Read the model definition and answer for the solid it produces. Units are mm, in the model's axes. Face numbers are marked on the shaded views. A direction names the side the tool comes from. Give positions to 0.01 mm unless a question says otherwise; leave off trailing zeros. Loops run counter-clockwise (first coordinate to the right, second up) from the corner with the lowest first, then second, coordinate; pieces in that order, holes last. Notation, with made-up numbers: (89, -24) - (146, -24) arc R22 cw to (146, 3) - close; hole circle Ø6 at (-26.75, -31). An arc over 180 degrees is marked (long way). Put each result on its own line as item: value. Start each with the question number.
1. A cutting plane is placed at B-B, the plane x = 10.25. Determine the outline of the cut face in (y, z).
2. Given pin 1 Ø5.5 at (x, y) = (-1, -1) entering from -Z; pin 2 Ø6 at (y, z) = (-3.5, -9) entering from +X; pin 3 Ø2 at (y, z) = (-6, -18.5) entering from +X, each flat-ended and moving along its own axis, determine where each tip first touches the part or whether it passes through.
3. A cutting plane is placed at A-A, the plane z = -3.25. Determine the outline of the cut face in (x, y), plus the area to 3 significant figures.
4. A cutting plane is placed at C-C, the plane z = -17.25. Determine the outline of the cut face in (x, y), plus the area to 3 significant figures.
5. Consider L1, parallel to Z at x = 6.25, y = -9.75; L2, parallel to Y at x = 0, z = 3; L3, parallel to Z at x = -5.5, y = 7.25. Determine where each line is inside the solid, lowest interval first. Write a range as from..to.
6. For the marked faces 1, 2 and 3, determine the directions among +Z, -Z, +X, -X, +Y, -Y from which every point of the face is accessible in a straight line to the end or side of a thin tool.
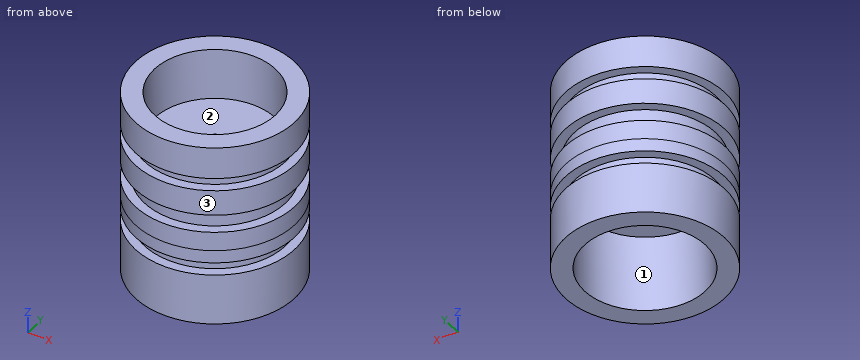
Autodesk Inventor part; units mm, degrees
ref_plane "Work Plane2" through (0, 0, -14) normal (0, 0, -1) x (-1, 0, 0)
ref_plane "Work Plane3" through (0, 0, 1.8) normal (0, 0, 1) x (1, 0, 0)
ref_plane "YZ Plane" through (0, 0, 0) normal (1, 0, 0) x (0, 1, 0)
sketch "Sketch1" plane through (0, 0, 0) normal (0, 0, 1) x (1, 0, 0)
  circle A0 centre (0, 0) radius 0.5
  circle A1 centre (0, 0) radius 8.1639
  point P0 (0, 0)
extrude "Extrusion1" add sketch "Sketch1" along normal blind 9.8
ref_plane "Work Plane1" through (0, 0, -10) normal (0, 0, 1) x (1, 0, 0)
sketch "Sketch2" plane through (0, 0, -10) normal (0, 0, 1) x (1, 0, 0)
  line L0 (5, 5) -> (-5, 5)
  arc A0 (-5, 5) -> (-6, 4) centre (-5, 4) ccw
  line L1 (-6, 4) -> (-6, -4)
  arc A1 (-6, -4) -> (-5, -5) centre (-5, -4) ccw
  line L2 (-5, -5) -> (5, -5)
  arc A2 (5, -5) -> (6, -4) centre (5, -4) ccw
  line L3 (6, -4) -> (6, 4)
  arc A3 (6, 4) -> (5, 5) centre (5, 4) ccw
  circle A4 centre (3.5, 2.5) radius 1.75
  circle A5 centre (-3.5, -2.5) radius 1.75
  circle A6 centre (4.5, 0) radius 0.625
  circle A7 centre (-4.5, 0) radius 0.625
  circle A8 centre (0, 0) radius 2
  line L4 (0, 0) -> (5.8769, -4.8974)
  line L5 (5.8769, -4.8974) -> (7.0292, -5.8577)
  circle A9 centre (0, 0) radius 9.15
  circle A10 centre (0, 0) radius 8.1639
  circle A11 centre (0, 0) radius 13.1
  line L6 (3.0438, -10.097) -> (-9.0477, 9.4736)
  line L7 (-6.9043, 6.0044) -> (-9.0477, 9.4736)
  line L8 (3.0438, -10.097) -> (-5, 4)
  line L9 (-5, 4) -> (-4.2491, 2.684)
  point P0 (0, 0)
  dimension "d3" = 26.2
  dimension "d2" = 1.5
  dimension "d4" = 18.3
extrude "Extrusion2" add sketch "Sketch2" against normal blind 9 contours A9 L8 L6 | A11
sketch "Sketch3" plane through (0, 0, -10) normal (0, 0, 1) x (1, 0, 0)
  arc A0 (0.8877, 1.2091) -> (1.103, -1.0166) centre (0, 0) ccw
  line L0 (0.8877, 1.2091) -> (1.103, -1.0166)
  circle A1 centre (0, 0) radius 13.1
  circle A2 centre (0, 0) radius 9.15
  circle A3 centre (0, 0) radius 8.1639
  circle A4 centre (0, 0) radius 0.5
  point P0 (0, 0)
extrude "Extrusion3" add sketch "Sketch3" along normal up to surface (19.8 mm away) contours A1 | A2 | A3
sketch "Sketch4" plane through (0, 0, 9.8) normal (0, 0, 1) x (1, 0, 0)
  circle A0 centre (0, 0) radius 13.1
  circle A1 centre (0, 0) radius 0.5
  point P0 (0, 0)
extrude "Extrusion4" add sketch "Sketch4" against normal blind 10 contours A1
sketch "Sketch5" plane through (0, 0, 9.8) normal (0, 0, 1) x (1, 0, 0)
  circle A0 centre (0, 0) radius 13.1
  point P0 (0, 0)
extrude "Extrusion5" add sketch "Sketch5" against normal up to surface (9.8 mm away)
sketch "Sketch6" plane through (0, 0, -0.2) normal (0, 0, -1) x (-1, 0, 0)
  circle A0 centre (0, 0) radius 0.5
  point P0 (0, 0)
extrude "Extrusion6" cut sketch "Sketch6" against normal up to surface (0.2 mm away)
sketch "Sketch8" plane through (0, 0, 9.8) normal (0, 0, 1) x (1, 0, 0)
  circle A0 centre (0, 0) radius 13.1
  point P0 (0, 0)
extrude "Extrusion7" cut sketch "Sketch8" against normal blind 3
sketch "Sketch10" plane through (0, 0, -19) normal (0, 0, -1) x (-1, 0, 0)
  circle A0 centre (0, 0) radius 13.1
  circle A1 centre (0, 0) radius 9.15
  circle A2 centre (0, 0) radius 12.5
  line L0 (-12.5, 0) -> (-9.15, 0)
  circle A3 centre (0, 0) radius 9.15
  line L1 (-9.15, 0) -> (-10.825, 0)
  circle A4 centre (0, 0) radius 10.825
  point P0 (0, 0)
  dimension "d18" = 25
extrude "Extrusion8" cut sketch "Sketch10" against normal up to surface (9 mm away)
extrude "Extrusion9" cut sketch "Sketch10" against normal through all contours A0
sketch "Sketch11" plane through (0, 0, -19) normal (0, 0, -1) x (-1, 0, 0)
  circle A0 centre (0, 0) radius 10.825
  line L0 (-0.8877, 1.2091) -> (-1.103, -1.0166)
  arc A1 (-1.103, -1.0166) -> (-0.8877, 1.2091) centre (0, 0) ccw
  circle A2 centre (0, 0) radius 10.825
  circle A3 centre (0, 0) radius 12.5
  line L1 (-12.5, 0) -> (-9.5, 0)
  circle A4 centre (0, 0) radius 9.5
  point P0 (0, 0)
  dimension "d23" = 3
extrude "Extrusion10" add sketch "Sketch11" against normal up to surface (9 mm away) contours A0
sketch "Sketch12" plane through (0, 0, 6.8) normal (0, 0, 1) x (1, 0, 0)
  circle A0 centre (0, 0) radius 12.5
  circle A1 centre (0, 0) radius 9.5
  line L0 (0.8877, 1.2091) -> (1.103, -1.0166)
  arc A2 (0.8877, 1.2091) -> (1.103, -1.0166) centre (0, 0) ccw
  point P0 (0, 0)
extrude "Extrusion11" cut sketch "Sketch12" against normal blind 8 contours A1 | L0 A2
sketch "Sketch13" plane through (0, 0, -1.2) normal (0, 0, 1) x (1, 0, 0)
  line L0 (1.103, -1.0166) -> (0.8877, 1.2091)
  arc A0 (0.8877, 1.2091) -> (1.103, -1.0166) centre (0, 0) ccw
  circle A1 centre (0, 0) radius 9.5
  circle A2 centre (0, 0) radius 11.0657
  circle A3 centre (0, 0) radius 9.5
  circle A4 centre (0, 0) radius 12.5
  point P0 (0, 0)
extrude "Extrusion12" cut sketch "Sketch13" against normal up to surface (8.8 mm away) contours A4
sketch "Sketch14" plane through (0, 0, -10) normal (0, 0, 1) x (1, 0, 0)
  circle A0 centre (0, 0) radius 11.0657
  circle A1 centre (0, 0) radius 12.5
  point P0 (0, 0)
extrude "Extrusion13" add sketch "Sketch14" along normal blind 3
sketch "Sketch15" plane through (0, 0, -1.2) normal (0, 0, -1) x (-1, 0, 0)
  circle A0 centre (0, 0) radius 12.5
  circle A1 centre (0, 0) radius 11.0657
  point P0 (0, 0)
extrude "Extrusion14" add sketch "Sketch15" along normal blind 3
ref_plane "Work Plane2" through (0, 0, -14) normal (0, 0, -1) x (-1, 0, 0)
ref_plane "Work Plane3" through (0, 0, 1.8) normal (0, 0, 1) x (1, 0, 0)
sketch "Sketch16" plane through (0, 0, -14) normal (0, 0, -1) x (-1, 0, 0)
  circle A0 centre (0, 0) radius 12.5
  circle A1 centre (0, 0) radius 11.0657
  point P0 (0, 0)
extrude "Extrusion15" cut sketch "Sketch16" against normal blind 2
sketch "Sketch17" plane through (0, 0, 1.8) normal (0, 0, 1) x (1, 0, 0)
  circle A0 centre (0, 0) radius 12.5
  circle A1 centre (0, 0) radius 11.0657
  point P0 (0, 0)
extrude "Extrusion16" cut sketch "Sketch17" against normal blind 2
sketch "Sketch18" plane through (0, 0, -19) normal (0, 0, -1) x (-1, 0, 0)
  circle A0 centre (0, 0) radius 9.5
  circle A1 centre (0, 0) radius 12.5
  point P0 (0, 0)
extrude "Extrusion17" add sketch "Sketch18" along normal blind 2
sketch "Sketch19" plane through (0, 0, -21) normal (0, 0, -1) x (-1, 0, 0)
  circle A0 centre (0, 0) radius 12.5
  circle A1 centre (0, 0) radius 9.5
  point P0 (0, 0)
extrude "Extrusion18" add sketch "Sketch19" along normal blind 1
properties part number "felga" material "Aluminum 6061"
Return value:
1. outline: (-7.15, -22) - (7.15, -22) - (7.15, -14) - (4.17, -14) - (4.17, -12) - (7.15, -12) - (7.15, -7) - (4.17, -7) - (4.17, -4.2) - (7.15, -4.2) - (7.15, -0.2) - (4.17, -0.2) - (4.17, 1.8) - (7.15, 1.8) - (7.15, 6.8) - (-7.15, 6.8) - (-7.15, 1.8) - (-4.17, 1.8) - (-4.17, -0.2) - (-7.15, -0.2) - (-7.15, -4.2) - (-4.17, -4.2) - (-4.17, -7) - (-7.15, -7) - (-7.15, -12) - (-4.17, -12) - (-4.17, -14) - (-7.15, -14) - close
2. pin 1: stops at z = -10
2. pin 2: stops at x = 12.49
2. pin 3: stops at x = 11.46
3. outline: circle Ø25 at (0, 0); hole (0.89, 1.21) arc R1.5 ccw (long way) to (1.1, -1.02) - close
3. area: 485 mm2
4. outline: circle Ø25 at (0, 0); hole circle Ø19 at (0, 0)
4. area: 207 mm2
5. L1: z = -22..-14, -12..-7, -4.2..-0.2, 1.8..6.8
5. L2: y = -12.5..-9.5, 9.5..12.5
5. L3: z = -10..-1.2
6. face 1: -Z
6. face 2: +Z
6. face 3: +Z, -Z
